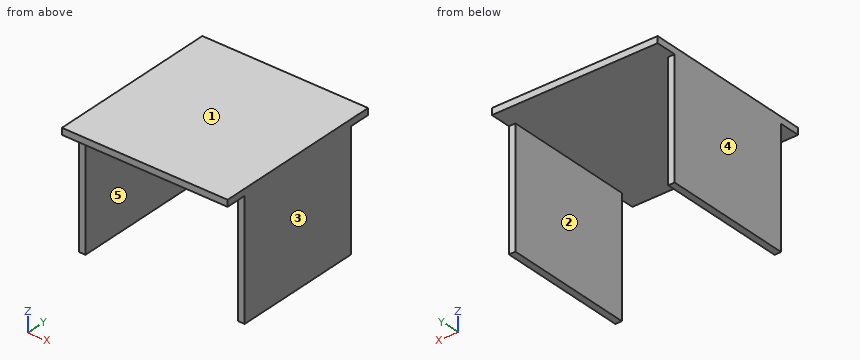
```python
from build123d import *

# Parameters (mm, degrees)
SKETCH006_W  = 10
SKETCH006_H  = 9.5
PAD002_DEPTH = 0.5
SKETCH007_W  = 12.7
SKETCH007_H  = 13.2
PAD003_DEPTH = 0.5
SKETCH008_W  = 10
SKETCH008_H  = 9.5
PAD004_DEPTH = 0.5


with BuildPart() as part:
    # Sketch006 → Pad002 (new body)
    with BuildSketch(Plane.YZ.offset(6.35)):
        with Locations((0, 4.75)):
            Rectangle(SKETCH006_W, SKETCH006_H)
    extrude(amount=-PAD002_DEPTH)

    # Sketch007 → Pad003 (join)
    with BuildSketch(Plane.XY.offset(9.5)):
        Rectangle(SKETCH007_W, SKETCH007_H)
    extrude(amount=-PAD003_DEPTH)

    # Sketch008 → Pad004 (join)
    with BuildSketch(Plane.YZ.offset(-6.35)):
        with Locations((0, 4.75)):
            Rectangle(SKETCH008_W, SKETCH008_H)
    extrude(amount=PAD004_DEPTH)


solid = part.part
```
Verification items for the finished model (mm, model axes). Face numbers are marked on the shaded views. A direction names the side the tool comes from. Coordinates: 2 decimals unless noted, no trailing zeros. Loops run counter-clockwise (first coordinate to the right, second up) from the corner with the lowest first, then second, coordinate; pieces in that order, holes last. Notation, with made-up numbers: (-18, -32) - (29, -32) arc R15 ccw to (29, -4) - close; hole circle Ø8 at (-35, 28.5). An arc over 180 degrees is marked (long way). Put each result on its own line as item: value.
Item 1: Draft check along X on the marked faces 1, 2 and 3. Enter one of: pulls with the +X half, pulls with the -X half, needs draft (parallel to the pull), parting line crosses it, or undercut.
Conclusion:
face 1: needs draft
face 2: undercut
face 3: pulls with the +X half
Item 2: Set-up check for the marked faces 4 and 5: record each of +Z, -Z, +X, -X, +Y, -Y from which the full face is reachable in a straight line by a thin tool's end or side.
Conclusion:
face 4: +Z, -Z, -X, +Y, -Y
face 5: -Z, +Y, -Y
Item 3: Gauge pin test, flat end, axial feed: pin 1 Ø0.6 at (x, z) = (6, 2.5) entering from -Y. Record the tip position at first contact, or that the pin passes through.
Conclusion:
pin 1: stops at y = -5
Item 4: Section check C-C (x = 3.5). Enter the section's corners in (y, z).
Conclusion:
outline: (-6.6, 9) - (6.6, 9) - (6.6, 9.5) - (-6.6, 9.5) - close
Item 5: Section check B-B (y = 4). Enter the section's corners in (x, z).
Conclusion:
outline: (-6.35, 0) - (-5.85, 0) - (-5.85, 9) - (5.85, 9) - (5.85, 0) - (6.35, 0) - (6.35, 9.5) - (-6.35, 9.5) - close
Item 6: Section check D-D (y = 5.5). Enter the section's corners in (x, z).
Conclusion:
outline: (-6.35, 9) - (6.35, 9) - (6.35, 9.5) - (-6.35, 9.5) - close
Item 7: Scan lines: line 1 along X through (y, z) = (-1, 8.5); line 2 along Z through (x, y) = (-2.25, 3.5). Record each from-to range of solid material in increasing order.
Conclusion:
line 1: x = -6.35 to -5.85, 5.85 to 6.35
line 2: z = 9 to 9.5
Item 8: Section check A-A (z = 4.5). Enter the section's corners in (x, y).
Conclusion:
outline: (-6.35, -5) - (-5.85, -5) - (-5.85, 5) - (-6.35, 5) - close; (5.85, -5) - (6.35, -5) - (6.35, 5) - (5.85, 5) - close
